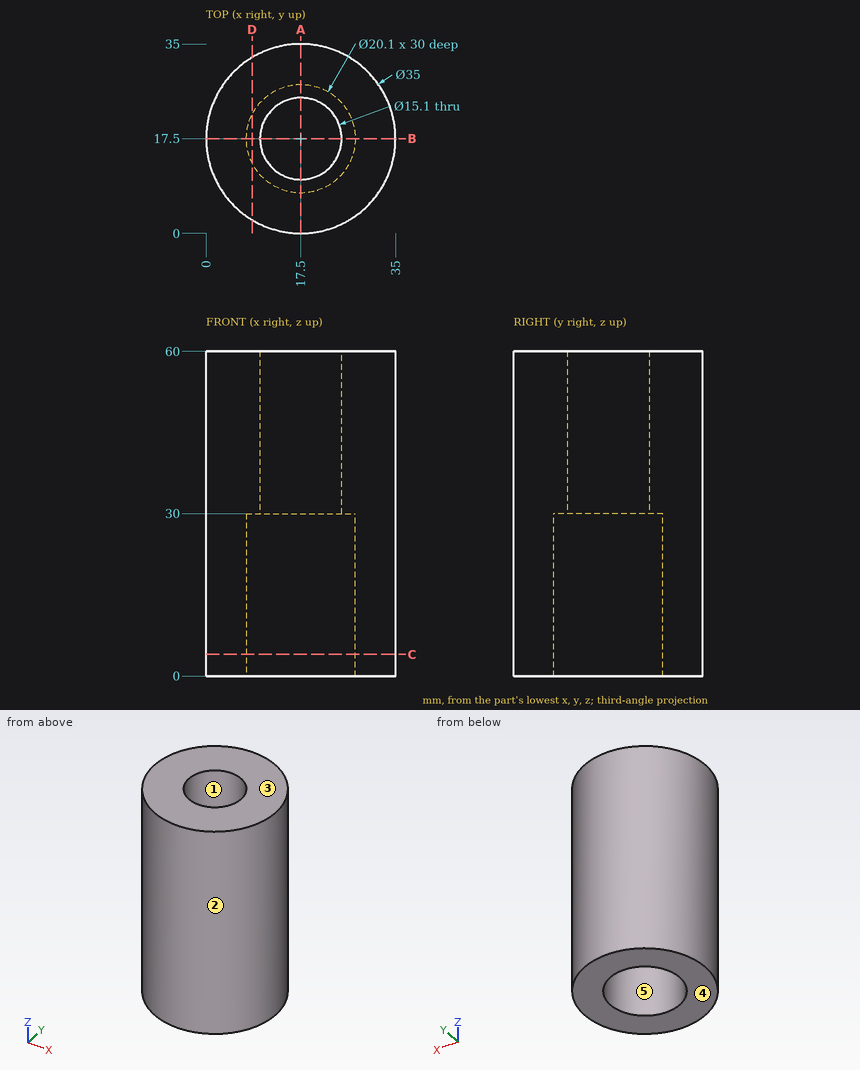
Drawing for the job (mm, zero at the part's lowest x, y, z). A direction names the side the tool comes from. Coordinates: 2 decimals unless noted, no trailing zeros. Write each loop counter-clockwise with the first axis right and the second up, starting at its lowest first coordinate (ties: lowest second). Pieces come first, ordered by that corner, then holes. Notation, with made-up numbers: (-3.5, -17) -> (18.5, -17) arc R27 ccw to (18.5, 10) -> close; hole circle Ø5 at (78.5, -34). An arc over 180 degrees is marked (long way). One line per item, written item: value. Start each with the question number.
1) Pull direction X, two halves, no side cores. Call the marked faces 1, 2 and 3: +X half, -X half, draft (parallel to the pull), parting line (faces both ways), or undercut.
2) Slice it at D-D on x = 8.5. Write the cut outline in (y, z), then the cut area to 3 significant figures.
3) Probe probe 1 along Y at (x, z) = (17, 20); probe 2 along X at (y, z) = (18, 37.5); probe 3 along X at (y, z) = (14, 5). List the from-to ranges inside material, lowest first.
4) Slice it at A-A on x = 17.5. Write the cut outline in (y, z), then the cut area to 3 significant figures.
5) Which spindle directions (+Z, -Z, +X, -X, +Y, -Y) get a long thin tool onto all of the face, cutting with end or side? Do the marked faces 4 and 5. Say none if no direction does.
6) Slice it at C-C on z = 4. Write the cut outline in (x, y).
7) Flat gauge pins, fed straight in: pin 1 Ø3 at (x, z) = (12, 52) entering from -Y; pin 2 Ø3 at (x, z) = (7.5, 37) entering from -Y; pin 3 Ø3 at (x, z) = (31, 20.5) entering from -Y. Where does each tip first touch, or does it go through?
Answers follow:
1. face 1: undercut
1. face 2: parting line
1. face 3: draft
2. outline: (2.49, 0) -> (13.03, 0) -> (13.03, 30) -> (21.97, 30) -> (21.97, 0) -> (32.51, 0) -> (32.51, 60) -> (2.49, 60) -> close
2. area: 1,530 mm2
3. probe 1: 0.01 to 7.46, 27.54 to 34.99
3. probe 2: 0.01 to 9.97, 25.03 to 34.99
3. probe 3: 0.35 to 8.08, 26.92 to 34.65
4. outline: (0, 0) -> (7.45, 0) -> (7.45, 30) -> (9.95, 30) -> (9.95, 60) -> (0, 60) -> close; (25.05, 30) -> (27.55, 30) -> (27.55, 0) -> (35, 0) -> (35, 60) -> (25.05, 60) -> close
4. area: 1,040 mm2
5. face 4: -Z, +X, -X, +Y, -Y
5. face 5: -Z
6. outline: circle Ø35 at (17.5, 17.5); hole circle Ø20.1 at (17.5, 17.5)
7. pin 1: y = 0.46
7. pin 2: y = 2.2
7. pin 3: y = 4.76
